Model file for the job. Use its own axes, mm. A direction names the side the tool comes from. Round coordinates to 2 decimals unless told otherwise and drop trailing zeros. Order: outer loops, then holes, each group sorted by start corner. A loop starts at its lowest first (then second) coordinate and runs counter-clockwise, first axis right, second up. Notation, with made-up numbers: (-9, 42.5) -> (9, 42.5) arc R12 ccw to (9, 59.5) -> close; hole circle Ø1 at (83, -9). An arc over 180 degrees is marked (long way). Use CSV: the item, a comma, the result in double quotes.
```python
from build123d import *

# Parameters (mm, degrees)
F0_R     = 5
F1_DEPTH = 40
F2_R     = 5
F4_DEPTH = 200
F3_R     = 10
F3_R_2   = 5
F5_DEPTH = 100


with BuildPart() as f1:
    # F0 (on Front) → F1 (new body)
    with BuildSketch(Plane.XZ):
        Circle(F0_R)
    extrude(amount=F1_DEPTH)

    # F2 (on face) → F4 (join)
    with BuildSketch(Plane.XZ.offset(40)):
        Circle(F2_R)
    extrude(amount=F4_DEPTH)

    # F3 (on face) → F5 (join)
    with BuildSketch(Plane.XZ.offset(40)):
        Circle(F3_R)
        Circle(F3_R_2, mode=Mode.SUBTRACT)
    extrude(amount=F5_DEPTH)


solid = f1.part
```
Q1. Probe line 1 along X through (y, z) = (-103, -0.75); line 2 along Y through (x, z) = (-5.25, 3); line 3 along X through (y, z) = (-202, -0.5). List the from-to ranges inside material, lowest first.
From the geometry:
line 1,"x = -9.97 to 9.97"
line 2,"y = -140 to -40"
line 3,"x = -4.97 to 4.97"
Q2. Cut at A-A (z = 0). Give the cut face in (x, y).
From the geometry:
outline,"(-10, -140) -> (-5, -140) -> (-5, -240) -> (5, -240) -> (5, -140) -> (10, -140) -> (10, -40) -> (5, -40) -> (5, 0) -> (-5, 0) -> (-5, -40) -> (-10, -40) -> close"
Q3. Which spindle directions (+Z, -Z, +X, -X, +Y, -Y) get a long thin tool onto all of the face, cutting with end or side? Do faces 1 (the cylindrical face through (-1.08, -19.72, -4.88)), 2 (the flat face through (0, -240, 0)), 3 (the cylindrical face through (-1.08, -189.3, -4.88)). Say none if no direction does.
From the geometry:
face 1,"+Y"
face 2,"+Z, -Z, +X, -X, -Y"
face 3,"-Y"
Q4. Cut at D-D (y = -175). Give the cut face in (x, z), plus the area to 3 significant figures.
From the geometry:
outline,"circle Ø10 at (0, 0)"
area,"78.5 mm²"
Q5. Cut at C-C (y = -104.5). Give the cut face in (x, z), plus the area to 3 significant figures.
From the geometry:
outline,"circle Ø20 at (0, 0)"
area,"314 mm²"
Q6. Pin check, flat tips, straight feed: pin 1 (2 mm diameter, centred on x = 1, y = -161.5, fed in from +Z); pin 2 (6 mm diameter, centred on x = -5, y = -89, fed in from +Z); pin 3 (12 mm diameter, centred on y = -190.5, z = -1, fed in from -X). Stop position of each tip, or through.
From the geometry:
pin 1,"stops at z = 5"
pin 2,"stops at z = 9.8"
pin 3,"stops at x = -5"
Q7. Cut at B-B (x = 0). Give the cut face in (y, z), plus the area to 3 significant figures.
From the geometry:
outline,"(-240, -5) -> (-140, -5) -> (-140, -10) -> (-40, -10) -> (-40, -5) -> (0, -5) -> (0, 5) -> (-40, 5) -> (-40, 10) -> (-140, 10) -> (-140, 5) -> (-240, 5) -> close"
area,"3,400 mm²"
